```python
from build123d import *

# Parameters (mm, degrees)
F1_DEPTH = 76.2
F2_R     = 9.525
F3_DEPTH = 38.101
F4_R     = 6.35
F5_DEPTH = 25.4
F6_DEPTH = 12.7


with BuildPart() as f1:
    # F0 (on Front) → F1 (new body)
    with BuildSketch(Plane.XZ):
        Polygon((0, 0.552274), (-38.1, 0.552274), (-38.1, -37.547726), (0, -37.547726), (0, -3.861072), align=None)
    extrude(amount=-F1_DEPTH)

    # F2 (on face) → F3 (cut, through all)
    with BuildSketch(Plane.XY.offset(0.552274)):
        with Locations((-19.05, 38.1)):
            Circle(F2_R)
    extrude(amount=-F3_DEPTH, mode=Mode.SUBTRACT)

    # F4 (on face) → F5 (join)
    with BuildSketch(Plane.XY.offset(0.552274)):
        with BuildLine():
            Line((0, 76.2), (0, 0))
            Line((0, 0), (63.5, 0))
            ThreePointArc((63.5, 0), (101.6, 38.1), (63.5, 76.2))
            Line((63.5, 76.2), (0, 76.2))
        make_face()
        with Locations((12.7, 19.05)):
            Circle(F4_R, mode=Mode.SUBTRACT)
        with Locations((63.5, 19.05)):
            Circle(F4_R, mode=Mode.SUBTRACT)
        with Locations((12.7, 57.15)):
            Circle(F4_R, mode=Mode.SUBTRACT)
        with Locations((63.5, 57.15)):
            Circle(F4_R, mode=Mode.SUBTRACT)
    extrude(amount=-F5_DEPTH)

    # F4 (on face) → F6 (cut)
    with BuildSketch(Plane.XY.offset(0.552274)):
        with BuildLine():
            Line((0, 76.2), (0, 0))
            Line((0, 0), (63.5, 0))
            ThreePointArc((63.5, 0), (101.6, 38.1), (63.5, 76.2))
            Line((63.5, 76.2), (0, 76.2))
        make_face()
        with Locations((12.7, 19.05)):
            Circle(F4_R, mode=Mode.SUBTRACT)
        with Locations((63.5, 19.05)):
            Circle(F4_R, mode=Mode.SUBTRACT)
        with Locations((12.7, 57.15)):
            Circle(F4_R, mode=Mode.SUBTRACT)
        with Locations((63.5, 57.15)):
            Circle(F4_R, mode=Mode.SUBTRACT)
    extrude(amount=-F6_DEPTH, mode=Mode.SUBTRACT)


solid = f1.part
```
Verification items for the finished model (mm, model axes). A direction names the side the tool comes from. Coordinates: 2 decimals unless noted, no trailing zeros. Order: outer loops, then holes, each group sorted by start corner. A loop starts at its lowest first (then second) coordinate and runs counter-clockwise, first axis right, second up. Notation, with made-up numbers: (35, 48) -> (70, 48) arc R24 ccw to (70, 84) -> close; hole circle Ø6 at (-15.75, 20). An arc over 180 degrees is marked (long way). Answer as CSV lines item,"result". Start each with the question number.
1) Set-up check for faces 1 (the face through (50, 39, -24.848)), 2 (the face through (2, 76.2, -18)), 3 (the face through (0, 39, -6)): record each of +Z, -Z, +X, -X, +Y, -Y from which the full face is reachable in a straight line by a thin tool's end or side.
2) Release check for a two-part mould opening along X. For faces 4 (the face through (-38.1, 38, -18)), 5 (the face through (62.12, 50.95, -18.41)), 6 (the face through (-24, 47, 0.552)) record: released by +X, released by -X, zero draft, split by the parting line, or undercut.
3) Cross-section at C-C, the plane z = -27. Record the boundary of the cut face in (x, y) (3 decimals), then the cut area to 3 significant figures.
4) Cross-section at A-A, the plane x = -19.05. Record the boundary of the cut face in (y, z) (3 decimals), then the cut area to 3 significant figures.
5) Cross-section at B-B, the plane y = 24. Record the boundary of the cut face in (x, z).
6) Material ranges on L1, parallel to Y at x = 63.5, z = -18.5; L2, parallel to X at y = 38, z = -8; L3, parallel to X at y = 56, z = -23 (3 decimals), recorded low to high. Write a range as [from, to].
7) Cross-section at D-D, the plane x = 12.7. Record the boundary of the cut face in (y, z), then the cut area to 3 significant figures.
8) Gauge pin test, flat ends, axial feed: pin 1 Ø7.5 at (x, y) = (12.7, 19.05) entering from +Z; pin 2 Ø14 at (y, z) = (45.5, -3) entering from +X; pin 3 Ø8 at (y, z) = (42, -28.5) entering from +X; pin 4 Ø2 at (y, z) = (66.5, -24.5) entering from +X. Record the tip position at first contact, or that the pin passes through.
Conclusion:
1,face 1,"-Z, +X, +Y, -Y"
1,face 2,"+Z, -Z, +X, -X, +Y"
1,face 3,"+Z, +X, +Y, -Y"
2,face 4,"released by -X"
2,face 5,"undercut"
2,face 6,"zero draft"
3,outline,"(-38.1, 0) -> (0, 0) -> (0, 76.2) -> (-38.1, 76.2) -> close; hole circle Ø19.05 at (-19.05, 38.1)"
3,area,"2,620 mm²"
4,outline,"(0, -37.548) -> (28.575, -37.548) -> (28.575, 0.552) -> (0, 0.552) -> close; (47.625, -37.548) -> (76.2, -37.548) -> (76.2, 0.552) -> (47.625, 0.552) -> close"
4,area,"2,180 mm²"
5,outline,"(-38.1, -37.55) -> (0, -37.55) -> (0, -24.85) -> (8.72, -24.85) -> (8.72, -12.15) -> (0, -12.15) -> (0, 0.55) -> (-38.1, 0.55) -> close; (16.68, -24.85) -> (59.52, -24.85) -> (59.52, -12.15) -> (16.68, -12.15) -> close; (67.48, -24.85) -> (98.89, -24.85) -> (98.89, -12.15) -> (67.48, -12.15) -> close"
6,L1,"y = [0, 12.7], [25.4, 50.8], [63.5, 76.2]"
6,L2,"x = [-38.1, -28.57], [-9.53, 0]"
6,L3,"x = [-38.1, 6.455], [18.945, 57.255], [69.745, 97.133]"
7,outline,"(0, -24.85) -> (12.7, -24.85) -> (12.7, -12.15) -> (0, -12.15) -> close; (25.4, -24.85) -> (50.8, -24.85) -> (50.8, -12.15) -> (25.4, -12.15) -> close; (63.5, -24.85) -> (76.2, -24.85) -> (76.2, -12.15) -> (63.5, -12.15) -> close"
7,area,"645 mm²"
8,pin 1,"passes through"
8,pin 2,"stops at x = 0"
8,pin 3,"stops at x = 101.53"
8,pin 4,"stops at x = 89.97"
